Source: CAD feature listing. Evaluate the final solid. Frame: model axes, mm. Face numbers are marked on the shaded views. Give positions to 0.01 mm unless a question says otherwise; leave off trailing zeros. Order: outer loops, then holes, each group sorted by start corner. A loop starts at its lowest first (then second) coordinate and runs counter-clockwise, first axis right, second up.
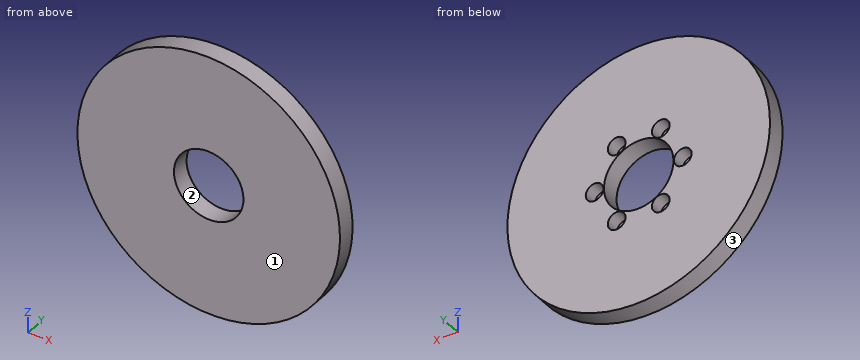
```python
from build123d import *

# Parameters (mm, degrees)
SKETCH1_R             = 85
BOSS_EXTRUDE1_DEPTH   = 12
SKETCH2_R             = 22.5
CUT_EXTRUDE1_DEPTH    = 121.805629008
SKETCH3_R             = 5.744458378
CUT_EXTRUDE2_DEPTH    = 8.640706
CIRPATTERN1_START     = 3.359294119
CIRPATTERN1_OUTLINE_R = 5.744458378
CIRPATTERN1_DEPTH     = 8.640705881


# Read off the part's stored shape, not the designer's step: CirPattern1
with BuildPart() as part:
    # Sketch1 → Boss-Extrude1 (new body)
    with BuildSketch(Plane(origin=(0, 0, 0), x_dir=(1, 0, 0), z_dir=(0, 1, 0))):
        with Locations(Location((0, 0, 0), (0, 0, 270))):
            Circle(SKETCH1_R)
    extrude(amount=BOSS_EXTRUDE1_DEPTH)

    # Sketch2 → Cut-Extrude1 (cut, through all)
    with BuildSketch(Plane(origin=(0, 0, 0), x_dir=(1, 0, 0), z_dir=(0, 1, 0))):
        with Locations(Location((0, 0, 0), (0, 0, 270))):
            Circle(SKETCH2_R)
    extrude(amount=CUT_EXTRUDE1_DEPTH, mode=Mode.SUBTRACT)

    # Sketch3 → Cut-Extrude2 (cut)
    with BuildSketch(Plane(origin=(0, 12, 0), x_dir=(1, 0, 0), z_dir=(0, 1, 0))):
        with Locations(Location((-28.560637046, 0, 0), (0, 0, 270))):
            Circle(SKETCH3_R)
    extrude(amount=-CUT_EXTRUDE2_DEPTH, mode=Mode.SUBTRACT)

    # CirPattern1 outline → CirPattern1 (cut)
    with BuildSketch(Plane(origin=(0, 0, 0), x_dir=(1, 0, 0), z_dir=(0, 1, 0)).offset(CIRPATTERN1_START)):
        with Locations((-14.280318523, -24.73423723)):
            Circle(CIRPATTERN1_OUTLINE_R)
        with Locations((14.280318523, -24.73423723)):
            Circle(CIRPATTERN1_OUTLINE_R)
        with Locations((28.560637046, 0)):
            Circle(CIRPATTERN1_OUTLINE_R)
        with Locations((14.280318523, 24.73423723)):
            Circle(CIRPATTERN1_OUTLINE_R)
        with Locations((-14.280318523, 24.73423723)):
            Circle(CIRPATTERN1_OUTLINE_R)
    extrude(amount=CIRPATTERN1_DEPTH, mode=Mode.SUBTRACT)


solid = part.part
```
1) Section query B-B, the plane z = 0. Return the cut outline in (x, y).
Report:
outline: (-85, 0) - (-22.5, 0) - (-22.5, 12) - (-22.82, 12) - (-22.82, 3.36) - (-34.31, 3.36) - (-34.31, 12) - (-85, 12) - close; (22.5, 0) - (85, 0) - (85, 12) - (34.31, 12) - (34.31, 3.36) - (22.82, 3.36) - (22.82, 12) - (22.5, 12) - close
2) Pin query (flat end, axial travel): pin 1 (5.5 mm diameter, centred on x = 29.5, z = 0, fed in from +Y); pin 2 (1 mm diameter, centred on x = -39.5, y = 5, fed in from -Z); pin 3 (1 mm diameter, centred on x = -12.5, y = 2, fed in from -Z). Return the tip coordinate at first contact, or that it passes through.
Report:
pin 1: stops at y = 3.36
pin 2: stops at z = -75.52
pin 3: stops at z = -84.15
3) Material intervals for L1, parallel to X at y = 7, z = 0; L2, parallel to X at y = 3.25, z = 0; L3, parallel to X at y = 7.5, z = 2.5, sorted ascending.
Report:
L1: x = -85 to -34.31, -22.82 to -22.5, 22.5 to 22.82, 34.31 to 85
L2: x = -85 to -22.5, 22.5 to 85
L3: x = -84.96 to -33.73, -23.39 to -22.36, 22.36 to 23.39, 33.73 to 84.96
4) Section query D-D, the plane z = -27.5. Return the cut outline in (x, y).
Report:
outline: (-80.43, 0) - (80.43, 0) - (80.43, 12) - (19.32, 12) - (19.32, 3.36) - (9.25, 3.36) - (9.25, 12) - (-9.25, 12) - (-9.25, 3.36) - (-19.32, 3.36) - (-19.32, 12) - (-80.43, 12) - close
5) Draft query along Z for the marked faces 1, 2 and 3. Return one class per face: +Z half, -Z half, draft (parallel to the pull), parting line (faces both ways), or undercut.
Report:
face 1: draft
face 2: undercut
face 3: parting line
6) Section query A-A, the plane x = 0. Return the cut outline in (y, z).
Report:
outline: (0, -85) - (12, -85) - (12, -22.5) - (0, -22.5) - close; (0, 22.5) - (12, 22.5) - (12, 85) - (0, 85) - close
7) Section query C-C, the plane y = 8.5. Return the cut outline in (x, z).
Report:
outline: circle Ø170 at (0, 0); hole circle Ø11.49 at (-28.56, 0); hole circle Ø45 at (0, 0); hole circle Ø11.49 at (-14.28, -24.73); hole circle Ø11.49 at (-14.28, 24.73); hole circle Ø11.49 at (14.28, -24.73); hole circle Ø11.49 at (14.28, 24.73); hole circle Ø11.49 at (28.56, 0)
